```python
from build123d import *

# Parameters (mm, degrees)
F1_DEPTH = 123.825
F2_W     = 9.525
F2_H     = 111.125
F3_DEPTH = 108.98632
F4_R     = 3.69316
F5_R     = 1.98374
F6_R     = 1.8288
F6_W     = 24
F6_H     = 9.5329248
F6_R_2   = 1.35255
F7_DEPTH = 248
F8_R     = 0.762


# Not quite as in the source:
# - an extrude ends at something that could not be found from the text; its depth is read off the source's solid


with BuildPart() as f1:
    # F0 (on Top) → F1 (new body)
    with BuildSketch(Plane.XY):
        Polygon((0, 16.27124), (0, 0), (-105.56748, 0), (-105.56748, 16.27124), (-107.2769, 16.27124), (-107.2769, -1.70942), (1.70942, -1.70942), (1.70942, 16.27124), align=None)
    extrude(amount=F1_DEPTH)

    # F2 (on face) → F3 (cut, through all)
    with BuildSketch(Plane.YZ.offset(1.70942)):
        with Locations((8.33374, 61.9125)):
            Rectangle(F2_W, F2_H)
    extrude(amount=-F3_DEPTH, mode=Mode.SUBTRACT)

    # F4
    f4_edges = [f1.edges().sort_by_distance(p)[0] for p in [
        (1.70942, -1.70942, 61.9125),
        (-107.2769, -1.70942, 61.9125),
    ]]
    fillet(f4_edges, radius=F4_R)

    # F5
    f5_edges = [f1.edges().sort_by_distance(p)[0] for p in [
        (0, 0, 61.9125),
        (-105.56748, 0, 61.9125),
    ]]
    fillet(f5_edges, radius=F5_R)

    # F6 (on face) → F7 (cut, through all)
    with BuildSketch(Plane.XZ.offset(1.70942)):
        with Locations((-52.78374, 120.65)):
            Circle(F6_R)
        with Locations((-5.15874, 120.65)):
            Circle(F6_R)
        with Locations((-100.40874, 120.65)):
            Circle(F6_R)
        with Locations((-45.63999, 3.175)):
            Circle(F6_R)
        with Locations((-59.92749, 3.175)):
            Circle(F6_R)
        with Locations((-89.99624, 111.9147876)):
            Rectangle(F6_W, F6_H)
        with Locations((-89.99624, 11.9102124)):
            Rectangle(F6_W, F6_H)
        with Locations((-15.57124, 111.9147876)):
            Rectangle(F6_W, F6_H)
        with Locations((-15.57124, 11.9102124)):
            Rectangle(F6_W, F6_H)
        with Locations((-98.02749, 96.7528672)):
            Circle(F6_R_2)
        with Locations((-98.02749, 27.0721328)):
            Circle(F6_R_2)
        with Locations((-7.53999, 27.0721328)):
            Circle(F6_R_2)
        with Locations((-7.53999, 96.7528672)):
            Circle(F6_R_2)
    extrude(amount=-F7_DEPTH, mode=Mode.SUBTRACT)

    # F8
    f8_edges = [f1.edges().sort_by_distance(p)[0] for p in [
        (-106.42219, 16.27124, 123.825),
        (0.85471, 16.27124, 123.825),
        (0.85471, 16.27124, 0),
        (-106.42219, 16.27124, 0),
    ]]
    fillet(f8_edges, radius=F8_R)


solid = f1.part
```
Part model, mm, in its own coordinate system. A direction names the side the tool comes from. Round coordinates to 2 decimals unless told otherwise and drop trailing zeros. Write each loop counter-clockwise with the first axis right and the second up, starting at its lowest first coordinate (ties: lowest second). Pieces come first, ordered by that corner, then holes.
Item 1: Cut at B-B, the plane z = 109. Give the cut face in (x, y), plus the area to 3 significant figures.
Results:
outline: (-107.28, 1.98) arc R3.69 ccw to (-103.58, -1.71) - (-102, -1.71) - (-102, 0) - (-103.58, 0) arc R1.98 cw to (-105.57, 1.98) - (-105.57, 3.57) - (-107.28, 3.57) - close; (-107.28, 13.1) - (-105.57, 13.1) - (-105.57, 16.27) - (-107.28, 16.27) - close; (-78, -1.71) - (-27.57, -1.71) - (-27.57, 0) - (-78, 0) - close; (-3.57, -1.71) - (-1.98, -1.71) arc R3.69 ccw to (1.71, 1.98) - (1.71, 3.57) - (0, 3.57) - (0, 1.98) arc R1.98 cw to (-1.98, 0) - (-3.57, 0) - close; (0, 13.1) - (1.71, 13.1) - (1.71, 16.27) - (0, 16.27) - close
area: 123 mm2
Item 2: Cut at C-C, the plane z = 23. Give the cut face in (x, y).
Results:
outline: (-107.28, 1.98) arc R3.69 ccw to (-103.58, -1.71) - (-1.98, -1.71) arc R3.69 ccw to (1.71, 1.98) - (1.71, 3.57) - (0, 3.57) - (0, 1.98) arc R1.98 cw to (-1.98, 0) - (-103.58, 0) arc R1.98 cw to (-105.57, 1.98) - (-105.57, 3.57) - (-107.28, 3.57) - close; (-107.28, 13.1) - (-105.57, 13.1) - (-105.57, 16.27) - (-107.28, 16.27) - close; (0, 13.1) - (1.71, 13.1) - (1.71, 16.27) - (0, 16.27) - close
Item 3: Probe L1, parallel to X at y = 14, z = 85; L2, parallel to Y at x = -69.5, z = 50; L3, parallel to X at y = 1.5, z = 102. List the from-to ranges inside material, lowest first.
Results:
L1: x = -107.28 to -105.57, 0 to 1.71
L2: y = -1.71 to 0
L3: x = -107.25 to -105.51, -0.06 to 1.68
Item 4: Which spindle directions (+Z, -Z, +X, -X, +Y, -Y) get a long thin tool onto all of the face, cutting with end or side? Do faces 4 (the flat face through (-105.567, 14, 47)), 5 (the cylindrical face through (-98.72, -0.87, 119.95)). Say none if no direction does.
Results:
face 4: +Z, -Z, +Y
face 5: +Y, -Y
Item 5: Two-plate mould, pull along Z, no slides. Class faces 1 (the cylindrical face through (-6.291, -0.867, 26.554)), 2 (the flat face through (-53, -1, 123.825)), 3 (the flat face through (-53, -1.709, 61)): +Z half, -Z half, draft (parallel to the pull), parting line (faces both ways), or undercut.
Results:
face 1: undercut
face 2: +Z half
face 3: draft
Item 6: Cut at A-A, the plane y = 5.25. Give the cut face in (x, z) (3 decimals), plus the area to 3 significant figures.
Results:
outline: (-107.277, 0) - (-105.567, 0) - (-105.567, 6.35) - (-107.277, 6.35) - close; (-107.277, 117.475) - (-105.567, 117.475) - (-105.567, 123.825) - (-107.277, 123.825) - close; (0, 0) - (1.709, 0) - (1.709, 6.35) - (0, 6.35) - close; (0, 117.475) - (1.709, 117.475) - (1.709, 123.825) - (0, 123.825) - close
area: 43.4 mm2
Item 7: Drop flat-ended pins along their axis: pin 1 Ø1.9 at (y, z) = (-1, 113) entering from +X; pin 2 Ø1.4 at (y, z) = (-1, 113) entering from -X; pin 3 Ø1.4 at (y, z) = (-0.5, 10.5) entering from +X; pin 4 Ø1.9 at (x, y) = (-88.5, -0.5) entering from -Z. Give the stop position or say it passes through.
Results:
pin 1: stops at x = 1.1
pin 2: stops at x = -106.49
pin 3: stops at x = 1.25
pin 4: stops at z = 0
